from build123d import *

# Parameters (mm, degrees)
SKETCH1_R           = 4.1275
BOSS_EXTRUDE1_DEPTH = 13.843
CUT_EXTRUDE1_DEPTH  = 21.463


with BuildPart() as part:
    # Sketch1 → Boss-Extrude1 (new body)
    with BuildSketch(Plane.XY):
        with BuildLine():
            Line((-2.174766514, 5.8293), (23.225233486, 5.8293))
            ThreePointArc((23.225233486, 5.8293), (39.256887261, -0.136207699), (47.489215864, -15.130538982))
            Line((47.489215864, -15.130538982), (48.675112128, -23.2029))
            add(Edge.make_bspline(
                [(46.212346009, -23.56470061), (45.056877099, -27.681849857), (51.170161996, -26.006789114), (48.675112128, -23.2029)],
                knots=[0, 0, 0, 0, 1, 1, 1, 1], degree=3))
            Line((46.212346009, -23.56470061), (45.055850098, -15.692466932))
            ThreePointArc((45.055850098, -15.692466932), (37.59061151, -2.592519956), (23.225233486, 1.98725211))
            Line((23.225233486, 1.98725211), (14.323446957, 1.98725211))
            ThreePointArc((14.323446957, 1.98725211), (8.536644874, 0.229383426), (4.70535824, -4.450191704))
            ThreePointArc((4.70535824, -4.450191704), (-8.359507137, -5.752383574), (-2.174766514, 5.8293))
        make_face()
        Circle(SKETCH1_R, mode=Mode.SUBTRACT)
    extrude(amount=BOSS_EXTRUDE1_DEPTH)

    # Sketch2 → Cut-Extrude1 (cut)
    with BuildSketch(Plane(origin=(0, 5.8293, 0), x_dir=(1, 0, 0), z_dir=(0, 1, 0))):
        with BuildLine():
            Line((4.276833486, -3.5814), (-9.616966514, -3.5814))
            Line((-9.616966514, -3.5814), (-9.616966514, -10.2616))
            Line((-9.616966514, -10.2616), (4.276833486, -10.2616))
            ThreePointArc((4.276833486, -10.2616), (7.616933486, -6.9215), (4.276833486, -3.5814))
        make_face()
    extrude(amount=-CUT_EXTRUDE1_DEPTH, mode=Mode.SUBTRACT)


solid = part.part
The model under review builds one solid part; all positions refer to its coordinate system, in mm. A direction names the side the tool comes from. Coordinates: 2 decimals unless noted, no trailing zeros. Loops run counter-clockwise (first coordinate to the right, second up) from the corner with the lowest first, then second, coordinate; pieces in that order, holes last. Notation, with made-up numbers: M 2,84.25 L 28,84.25 A26 cw 28,106.25 Z; hole C 87,82 d8. An arc over 180 degrees is marked long. Put each result on its own line as item: value. Start each with the question number.
Q1. Add section A-A (y = 0). Write out the cut boundary in (x, z), and give its area (3 significant figures).
Q2. The part is to be moulded in two halves that separate along Z. For faces 4 (the flat face through (16, 3, 0)), 5 (the flat face through (48.074, -19.11, 6.825)), 6 (the flat face through (-4, -2, 3.581)), say which applies: +Z half, -Z half, draft (parallel to the pull), parting line (faces both ways), or undercut.
Q3. Add section C-C (x = 0). Write out the cut boundary in (y, z).
Q4. Wall thickness on line 1 (X direction, y = 0, z = 11.1); line 2 (Z direction, x = -1, y = -8); line 3 (X direction, y = -3.5, z = 2): over which ranges is each line inside the solid? List them lowest first.
Q5. Add section D-D (y = -13). Write out the cut boundary in (x, z).
Q6. Add section B-B (x = 6). Write out the cut boundary in (y, z).
Q7. Clearance check with flat-ended pins moving along their axes: pin 1 (6 mm diameter, centred on x = 33, z = 9.5, fed in from +Y) (3 decimals); pin 2 (2 mm diameter, centred on x = 20.5, z = 4.5, fed in from -Y); pin 3 (6.5 mm diameter, centred on x = 0, y = 0, fed in from -Z); pin 4 (1.5 mm diameter, centred on x = 37.5, z = 3, fed in from +Y). State where each tip first meets the part, or that it passes through.
Q8. For faces 1 (the flat face through (19, 1.987, 7)), 2 (the flat face through (13, 5.829, 7)), 3 (the flat face through (-4, -2, 10.262)), list the 3-axis set-ups (+Z, -Z, +X, -X, +Y, -Y) from which the entire face can be reached by the end or side of a thin tool; tool diameter is ignored.
Answers:
1. outline: M -9.44,0 L -4.13,0 L -4.13,3.58 L -9.44,3.58 Z; M -9.44,10.26 L -4.13,10.26 L -4.13,13.84 L -9.44,13.84 Z; M 4.13,0 L 8.21,0 L 8.21,13.84 L 4.13,13.84 L 4.13,10.26 L 4.28,10.26 A3.34 cw 4.28,3.58 L 4.13,3.58 Z; M 33.49,0 L 39.1,0 L 39.1,13.84 L 33.49,13.84 Z
1. area: 154 mm^2
2. face 4: -Z half
2. face 5: draft
2. face 6: undercut
3. outline: M -8.73,0 L -4.13,0 L -4.13,3.58 L -8.73,3.58 Z; M -8.73,10.26 L -4.13,10.26 L -4.13,13.84 L -8.73,13.84 Z; M 4.13,0 L 5.83,0 L 5.83,3.58 L 4.13,3.58 Z; M 4.13,10.26 L 5.83,10.26 L 5.83,13.84 L 4.13,13.84 Z
4. line 1: x = -9.44 to -4.13, 4.13 to 8.21, 33.49 to 39.1
4. line 2: z = 0 to 3.58, 10.26 to 13.84
4. line 3: x = -9.37 to -2.19, 2.19 to 5.15, 38.64 to 42.48
5. outline: M 44.48,0 L 47.08,0 L 47.08,13.84 L 44.48,13.84 Z
6. outline: M -2.17,0 L 5.83,0 L 5.83,4.06 L -2.17,4.06 Z; M -2.17,9.78 L 5.83,9.78 L 5.83,13.84 L -2.17,13.84 Z
7. pin 1: stops at y = 4.875
7. pin 2: stops at y = 1.99
7. pin 3: passes through
7. pin 4: stops at y = 1.76
8. face 1: +Z, -Z, -Y
8. face 2: +Z, -Z, +X, -X, +Y
8. face 3: -X, +Y, -Y
